```python
from build123d import *

# Parameters (mm, degrees)
SKETCH1_W           = 12
SKETCH1_H           = 12
BOSS_EXTRUDE1_DEPTH = 70
CHAMFER1_SIZE       = 0.2
CHAMFER2_SIZE       = 1.5
SKETCH2_R           = 4
CUT_EXTRUDE1_DEPTH  = 72.274118725
TAP1_REACH          = 73.274
TAP1_BORE_R         = 1.621


with BuildPart() as part:
    # Sketch1 → Boss-Extrude1 (new body)
    with BuildSketch(Plane(origin=(0, 0, 0), x_dir=(1, 0, 0), z_dir=(0, 1, 0))):
        with Locations((6, 0)):
            Rectangle(SKETCH1_W, SKETCH1_H)
    extrude(amount=BOSS_EXTRUDE1_DEPTH)

    # Chamfer1
    chamfer1_edges = [part.edges().sort_by_distance(p)[0] for p in [
        (0, 35, 6),
        (0, 35, -6),
    ]]
    chamfer(chamfer1_edges, length=CHAMFER1_SIZE)

    # Chamfer2
    chamfer2_edges = [part.edges().sort_by_distance(p)[0] for p in [
        (12, 35, -6),
        (12, 35, 6),
    ]]
    chamfer(chamfer2_edges, length=CHAMFER2_SIZE)

    # Sketch2 → Cut-Extrude1 (cut, through all)
    with BuildSketch(Plane(origin=(0, 0, 0), x_dir=(0, 0, -1), z_dir=(1, 0, 0))):
        with Locations(Location((0, 62, 0), (0, 0, 180))):
            Circle(SKETCH2_R)
    extrude(amount=CUT_EXTRUDE1_DEPTH, mode=Mode.SUBTRACT)

    # Tap1 bore → Tap1 (cut, up to next)
    with BuildSketch(Plane(origin=(0, 70, 0), x_dir=(1, 0, 0), z_dir=(0, 1, 0)), mode=Mode.PRIVATE) as tap1_sk1:
        with Locations((8, 0)):
            Circle(TAP1_BORE_R)
    tap1_tool1 = extrude(tap1_sk1.sketch, amount=-TAP1_REACH, mode=Mode.PRIVATE) & part.part
    add(tap1_tool1.solids().sort_by_distance((8, 70, 0))[0], mode=Mode.SUBTRACT)


solid = part.part
```
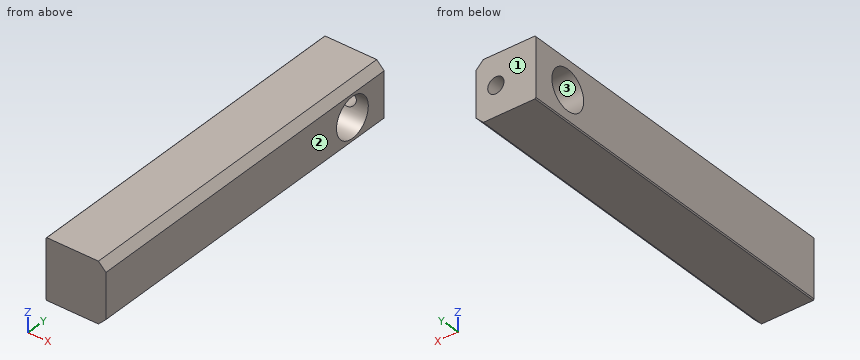
Work out the finished part from the listing and answer in its coordinate system (mm). Face numbers are marked on the shaded views. Round coordinates to 2 decimals unless told otherwise and drop trailing zeros. Write each loop counter-clockwise with the first axis right and the second up, starting at its lowest first coordinate (ties: lowest second). Pieces come first, ordered by that corner, then holes.
1) A cutting plane is placed at A-A on z = 0. Determine the outline of the cut face in (x, y).
2) Consider probe 1 along Z at (x, y) = (8, 68.6); probe 2 along Z at (x, y) = (3, 62); probe 3 along Y at (x, z) = (6.25, -0.25). Determine where each line is inside the solid, lowest interval first.
3) A cutting plane is placed at C-C on x = 2.5. Determine the outline of the cut face in (y, z), and give its area (3 significant figures).
4) A cutting plane is placed at B-B on y = 62. Determine the outline of the cut face in (x, z).
5) A flat-ended cylindrical pin translates along its axis: P1, Ø1.5, axis at x = 8.5, z = -1.5, coming from the +Y side. Find the tip coordinate at first contact, or state that the pin passes through.
6) A cutting plane is placed at D-D on y = 10.5. Determine the outline of the cut face in (x, z), and give its area (3 significant figures).
7) Determine the mould class of the marked faces 1, 2 and 3 for opening direction Y: pulls with the +Y half, pulls with the -Y half, needs draft (parallel to the pull), parting line crosses it, or undercut.
Entries:
1. outline: (0, 0) - (12, 0) - (12, 58) - (0, 58) - close; (0, 66) - (6.38, 66) - (6.38, 70) - (0, 70) - close; (9.62, 66) - (12, 66) - (12, 70) - (9.62, 70) - close
2. probe 1: z = -6 to -1.62, 1.62 to 6
2. probe 2: z = -6 to -4, 4 to 6
2. probe 3: y = 0 to 58.01, 65.99 to 70
3. outline: (0, -6) - (70, -6) - (70, 6) - (0, 6) - close; hole circle Ø8 at (62, 0)
3. area: 790 mm2
4. outline: (0, -5.8) - (0.2, -6) - (10.5, -6) - (12, -4.5) - (12, -4) - (0, -4) - close; (0, 4) - (12, 4) - (12, 4.5) - (10.5, 6) - (0.2, 6) - (0, 5.8) - close
5. P1: stops at y = 70
6. outline: (0, -5.8) - (0.2, -6) - (10.5, -6) - (12, -4.5) - (12, 4.5) - (10.5, 6) - (0.2, 6) - (0, 5.8) - close
6. area: 142 mm2
7. face 1: pulls with the +Y half
7. face 2: needs draft
7. face 3: undercut
